Check sheet for the modelled part. Datum: model origin and axes. Units: mm. Face numbers are marked on the shaded views. A direction names the side the tool comes from. Give positions to 0.01 mm unless a question says otherwise; leave off trailing zeros. Write each loop counter-clockwise with the first axis right and the second up, starting at its lowest first coordinate (ties: lowest second). Pieces come first, ordered by that corner, then holes. Notation, with made-up numbers: (81.5, -12) -> (128.5, -12) arc R16 cw to (128.5, 10) -> close; hole circle Ø4 at (23.5, 85). An arc over 180 degrees is marked (long way). Answer as a JSON object with one key per item and string values.
from build123d import *

# Parameters (mm, degrees)
SKETCH1_R           = 15
SKETCH1_R_2         = 12.5
BOSS_EXTRUDE1_DEPTH = 20
SKETCH2_R           = 15
BOSS_EXTRUDE2_DEPTH = 4
SKETCH3_W           = 12
SKETCH3_H           = 8
CUT_EXTRUDE1_DEPTH  = 4
SKETCH4_W           = 10
SKETCH4_H           = 10
BOSS_EXTRUDE3_DEPTH = 10
CUT_EXTRUDE2_DEPTH  = 7.5


with BuildPart() as part:
    # Sketch1 → Boss-Extrude1 (new body)
    with BuildSketch(Plane(origin=(0, 0, 0), x_dir=(1, 0, 0), z_dir=(0, 1, 0))):
        with Locations(Location((0, 0, 0), (0, 0, 270))):
            Circle(SKETCH1_R)
        with Locations(Location((0, 0, 0), (0, 0, 270))):
            Circle(SKETCH1_R_2, mode=Mode.SUBTRACT)
    extrude(amount=BOSS_EXTRUDE1_DEPTH)

    # Sketch2 → Boss-Extrude2 (add)
    with BuildSketch(Plane(origin=(0, 20, 0), x_dir=(1, 0, 0), z_dir=(0, 1, 0))):
        with Locations(Location((0, 0, 0), (0, 0, 270))):
            Circle(SKETCH2_R)
    extrude(amount=BOSS_EXTRUDE2_DEPTH)

    # Sketch3 → Cut-Extrude1 (cut)
    with BuildSketch(Plane(origin=(15, 0, 0), x_dir=(0, 0, -1), z_dir=(1, 0, 0))):
        with Locations((0, 4)):
            Rectangle(SKETCH3_W, SKETCH3_H)
    extrude(amount=-CUT_EXTRUDE1_DEPTH, mode=Mode.SUBTRACT)

    # Sketch4 → Boss-Extrude3 (add)
    with BuildSketch(Plane(origin=(0, 24, 0), x_dir=(1, 0, 0), z_dir=(0, 1, 0))):
        Rectangle(SKETCH4_W, SKETCH4_H)
    extrude(amount=BOSS_EXTRUDE3_DEPTH)

    # Sketch6 → Cut-Extrude2 (cut)
    with BuildSketch(Plane(origin=(0, 0, -5), x_dir=(-1, 0, 0), z_dir=(0, 0, -1))):
        with BuildLine():
            Line((-1.758355149, 34), (-3.758355149, 34))
            Line((-3.758355149, 34), (-3.758355149, 24))
            Line((-3.758355149, 24), (3.541644851, 24))
            Line((3.541644851, 24), (3.541644851, 24.674283625))
            Line((3.541644851, 24.674283625), (1.891753796, 25.274794859))
            ThreePointArc((1.891753796, 25.274794859), (1.811908661, 25.336062186), (1.781644851, 25.432046729))
            Line((1.781644851, 25.432046729), (1.781644851, 25.755508896))
            ThreePointArc((1.781644851, 25.755508896), (1.811908661, 25.85149344), (1.891753796, 25.912760766))
            Line((1.891753796, 25.912760766), (3.541644851, 26.513272))
            Line((3.541644851, 26.513272), (3.541644851, 27.187555625))
            Line((3.541644851, 27.187555625), (1.891753796, 27.788066859))
            ThreePointArc((1.891753796, 27.788066859), (1.811908661, 27.849334186), (1.781644851, 27.945318729))
            Line((1.781644851, 27.945318729), (1.781644851, 28.268780896))
            ThreePointArc((1.781644851, 28.268780896), (1.811908661, 28.36476544), (1.891753796, 28.426032766))
            Line((1.891753796, 28.426032766), (3.541644851, 29.026544))
            Line((3.541644851, 29.026544), (3.541644851, 29.700827625))
            Line((3.541644851, 29.700827625), (1.891753796, 30.301338859))
            ThreePointArc((1.891753796, 30.301338859), (1.811908661, 30.362606186), (1.781644851, 30.458590729))
            Line((1.781644851, 30.458590729), (1.781644851, 30.782052896))
            ThreePointArc((1.781644851, 30.782052896), (1.811908661, 30.87803744), (1.891753796, 30.939304766))
            Line((1.891753796, 30.939304766), (3.541644851, 31.539816))
            Line((3.541644851, 31.539816), (3.541644851, 32.214099625))
            Line((3.541644851, 32.214099625), (1.891753796, 32.814610859))
            ThreePointArc((1.891753796, 32.814610859), (1.811908661, 32.875878186), (1.781644851, 32.971862729))
            Line((1.781644851, 32.971862729), (1.781644851, 33.295324896))
            ThreePointArc((1.781644851, 33.295324896), (1.811908661, 33.39130944), (1.891753796, 33.452576766))
            Line((1.891753796, 33.452576766), (3.39578677, 34))
            Line((3.39578677, 34), (0.241644851, 34))
            Line((0.241644851, 34), (-1.758355149, 34))
        make_face()
    extrude(amount=-CUT_EXTRUDE2_DEPTH, mode=Mode.SUBTRACT)


solid = part.part
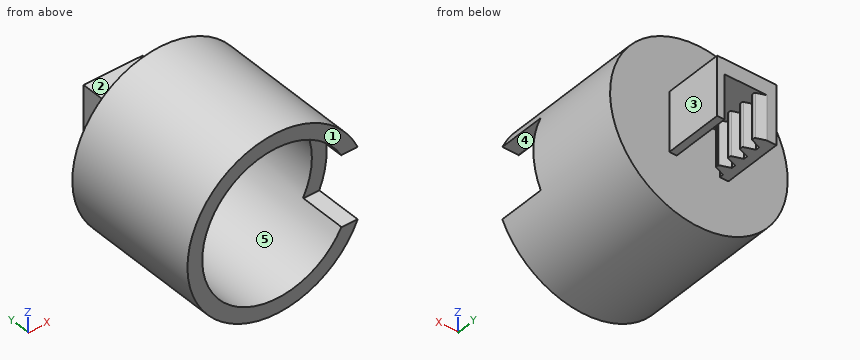
1. Sectioned sample at B-B, the plane x = 0. Enter the section's corners in (y, z).
Determined:
{"outline": "(0, -15) -> (24, -15) -> (24, 2.5) -> (34, 2.5) -> (34, 5) -> (24, 5) -> (24, 15) -> (0, 15) -> (0, 12.5) -> (20, 12.5) -> (20, -12.5) -> (0, -12.5) -> close"}
2. Sectioned sample at D-D, the plane y = 6. Enter the section's corners in (x, z), plus the area to 3 significant figures.
Determined:
{"outline": "(11, -6) -> (11, -5.94) arc R12.5 cw (long way) to (11, 5.94) -> (11, 6) -> (13.75, 6) arc R15 ccw (long way) to (13.75, -6) -> close", "area": "185 mm^2"}
3. Access from +Z, -Z, +X, -X, +Y, -Y to the whole of each face (thin tool, end or side, straight path). Record for the marked faces 1 and 2.
Determined:
{"face 1": "+Z, -Z, +X, -X, -Y", "face 2": "+Z, +X, -X, +Y"}
4. Go/stop test with flat-tipped pins: P1, Ø2, axis at x = 12.5, y = 2.5, coming from the -Z side; P2, Ø8, axis at x = 1.5, y = 31, coming from the -Z side; P3, Ø1, axis at x = 7, y = 26.5, coming from the +Z side; P4, Ø0.5, axis at y = 24.5, z = -2.5, coming from the +X side. Record where each tip stops, or that it passes through.
Determined:
{"P1": "z = -9.63", "P2": "z = -5", "P3": "through", "P4": "x = 5"}
5. Sectioned sample at C-C, the plane z = 3.5. Enter the section's corners in (x, y).
Determined:
{"outline": "(-14.59, 0) -> (-12, 0) -> (-12, 20) -> (12, 20) -> (12, 8) -> (14.59, 8) -> (14.59, 24) -> (5, 24) -> (5, 34) -> (-5, 34) -> (-5, 24) -> (-14.59, 24) -> close"}
6. Sectioned sample at A-A, the plane y = 15. Enter the section's corners in (x, z), plus the area to 3 significant figures.
Determined:
{"outline": "circle Ø30 at (0, 0); hole circle Ø25 at (0, 0)", "area": "216 mm^2"}
7. Mould release check, pull along X, two halves, no side actions. Record for the marked faces 3, 4 and 5: released by +X, released by -X, zero draft, split by the parting line, or undercut.
Determined:
{"face 3": "released by +X", "face 4": "zero draft", "face 5": "undercut"}
8. Scan lines: L1, parallel to Z at x = 0, y = 9; L2, parallel to Y at x = -2.5, z = 1.5. Record each from-to range of solid material in increasing order. Write a range as [from, to].
Determined:
{"L1": "[-15, -12.5], [12.5, 15]", "L2": "[20, 24], [25.05, 26.13], [27.57, 28.65], [30.08, 31.16], [32.59, 33.67]"}
